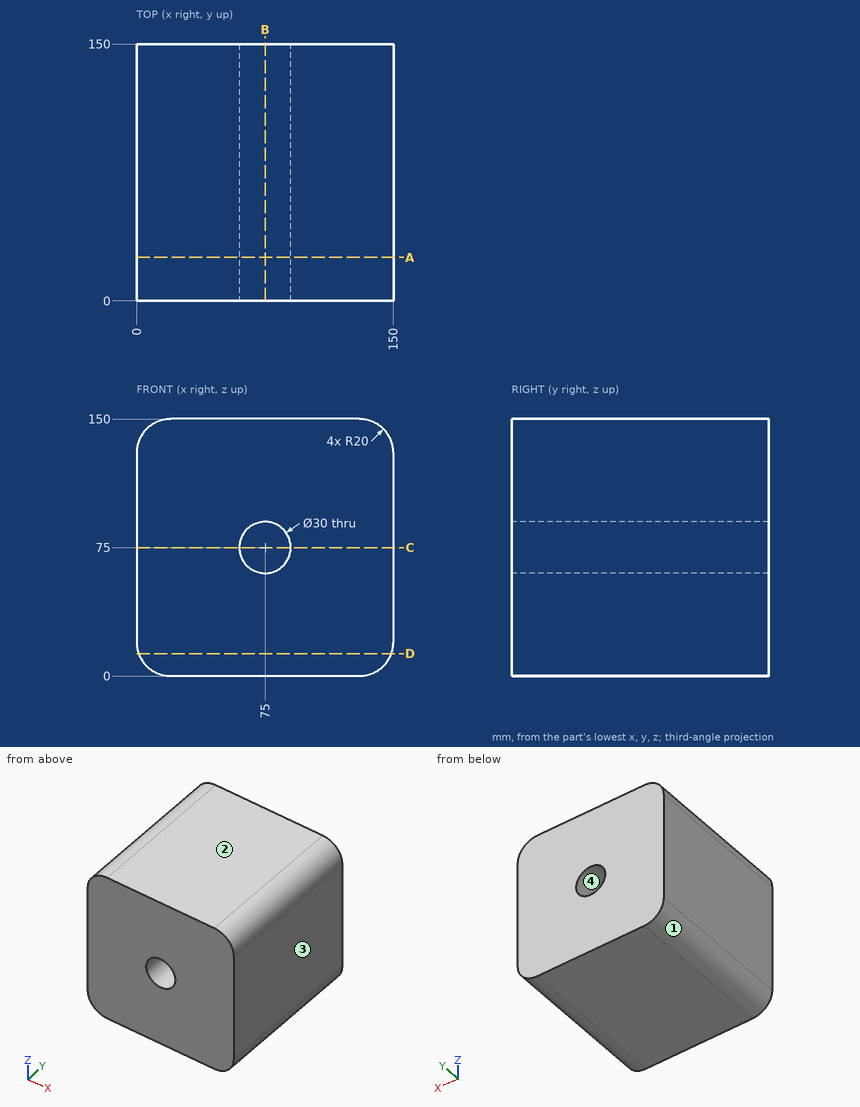
Source: three-view drawing plus pictorial views. Frame: mm from the lowest corner of the part. Give positions to 0.01 mm unless a question says otherwise; leave off trailing zeros. Order: outer loops, then holes, each group sorted by start corner. A loop starts at its lowest first (then second) coordinate and runs counter-clockwise, first axis right, second up. Notation, with made-up numbers: M -16.5,4.5 L 25.5,4.5 A12 ccw 25.5,18.5 Z; hole C 87.25,54 d3. An arc over 180 degrees is marked long. One line per question, with ' | ' between items. Start each with the question number.
1. Pull-direction query (X, two-part tool) for the marked faces 1, 2, 3 and 4; classes: released by +X, released by -X, zero draft, split by the parting line, or undercut.
2. Section query C-C (z = 75). Return the cut outline in (x, y), and give its area (3 significant figures).
3. First-contact query: pin 1 Ø8 at (x, y) = (134.5, 19) entering from +Z. Flat tip, straight axial feed; report the tip coordinate or a pass-through.
4. Section query B-B (x = 75). Return the cut outline in (y, z), and give its area (3 significant figures).
5. Section query D-D (z = 13). Return the cut outline in (x, y) (3 decimals), and give its area (3 significant figures).
6. Section query A-A (y = 25.5). Return the cut outline in (x, z), and give its area (3 significant figures).
7. Material intervals for probe 1 along Z at (x, y) = (75, 39.5); probe 2 along Z at (x, y) = (73, 22); probe 3 along X at (y, z) = (16, 79.5), sorted ascending. Write a range as [from, to].
Here are the results:
1) face 1: released by -X | face 2: zero draft | face 3: released by +X | face 4: undercut
2) outline: M 0,0 L 60,0 L 60,150 L 0,150 Z; M 90,0 L 150,0 L 150,150 L 90,150 Z | area: 18,000 mm²
3) pin 1: z = 149.99
4) outline: M 0,0 L 150,0 L 150,60 L 0,60 Z; M 0,90 L 150,90 L 150,150 L 0,150 Z | area: 18,000 mm²
5) outline: M 1.265,0 L 148.735,0 L 148.735,150 L 1.265,150 Z | area: 22,100 mm²
6) outline: M 0,20 A20 ccw 20,0 L 130,0 A20 ccw 150,20 L 150,130 A20 ccw 130,150 L 20,150 A20 ccw 0,130 Z; hole C 75,75 d30 | area: 21,400 mm²
7) probe 1: [0, 60], [90, 150] | probe 2: [0, 60.13], [89.87, 150] | probe 3: [0, 60.69], [89.31, 150]
